The listing builds one solid part. Answer for the finished solid, in the listing's coordinates (mm). A direction names the side the tool comes from. Give positions to 0.01 mm unless a question says otherwise; leave off trailing zeros. Write each loop counter-clockwise with the first axis right and the second up, starting at its lowest first coordinate (ties: lowest second). Pieces come first, ordered by that corner, then holes. Notation, with made-up numbers: (61, 21) -> (78, 21) arc R29 cw to (78, 52) -> close; hole circle Ø10 at (-31.75, -18). An arc over 180 degrees is marked (long way). One line per question, with ' | ' between items.
from build123d import *

# Parameters (mm, degrees)
SKETCH1_W           = 35
SKETCH1_H           = 35
SKETCH1_W_2         = 31
SKETCH1_H_2         = 31
BOSS_EXTRUDE1_DEPTH = 360
SKETCH2_R           = 4
CUT_EXTRUDE1_DEPTH  = 364.386846212


with BuildPart() as part:
    # Sketch1 → Boss-Extrude1 (new body)
    with BuildSketch(Plane(origin=(0, 0, 0), x_dir=(0, 0, -1), z_dir=(1, 0, 0))):
        with Locations((17.5, 17.5)):
            Rectangle(SKETCH1_W, SKETCH1_H)
        with Locations((17.5, 17.5)):
            Rectangle(SKETCH1_W_2, SKETCH1_H_2, mode=Mode.SUBTRACT)
    extrude(amount=BOSS_EXTRUDE1_DEPTH)

    # Sketch2 → Cut-Extrude1 (cut, through all)
    with BuildSketch(Plane.XY):
        with Locations((330, 17.5)):
            Circle(SKETCH2_R)
        with Locations((230, 17.5)):
            Circle(SKETCH2_R)
    extrude(amount=-CUT_EXTRUDE1_DEPTH, mode=Mode.SUBTRACT)


solid = part.part
Item 1: Determine the mould class of faces 1 (the face through (177, 33, -17)), 2 (the face through (177, 17, -35)), 3 (the face through (226.004, 17.676, -33.986)), 4 (the face through (177, 0, -17)) for opening direction Y: pulls with the +Y half, pulls with the -Y half, needs draft (parallel to the pull), parting line crosses it, or undercut.
Answers below:
face 1: undercut | face 2: needs draft | face 3: undercut | face 4: pulls with the -Y half
Item 2: Consider line 1 (Z direction, x = 339, y = 9); line 2 (Y direction, x = 195.5, z = -30.5); line 3 (X direction, y = 17, z = -1). Determine where each line is inside the solid, lowest interval first. Write a range as [from, to].
Answers below:
line 1: [-35, -33], [-2, 0] | line 2: [0, 2], [33, 35] | line 3: [0, 226.03], [233.97, 326.03], [333.97, 360]
Item 3: Find section D-D (x = 230). Write down the section's boundary in (y, z), then the cut area to 3 significant figures.
Answers below:
outline: (0, -35) -> (13.5, -35) -> (13.5, -33) -> (2, -33) -> (2, -2) -> (13.5, -2) -> (13.5, 0) -> (0, 0) -> close; (21.5, -35) -> (35, -35) -> (35, 0) -> (21.5, 0) -> (21.5, -2) -> (33, -2) -> (33, -33) -> (21.5, -33) -> close | area: 232 mm²
Item 4: A flat-ended cylindrical pin translates along its axis: pin 1 (5 mm diameter, centred on x = 230, y = 17.5, fed in from -Z). Find the tip coordinate at first contact, or state that the pin passes through.
Answers below:
pin 1: through
Item 5: Find section C-C (x = 49). Write down the section's boundary in (y, z), then the cut area to 3 significant figures.
Answers below:
outline: (0, -35) -> (35, -35) -> (35, 0) -> (0, 0) -> close; hole (2, -33) -> (33, -33) -> (33, -2) -> (2, -2) -> close | area: 264 mm²
Item 6: Find section B-B (y = 25.5). Write down the section's boundary in (x, z).
Answers below:
outline: (0, -35) -> (360, -35) -> (360, -33) -> (0, -33) -> close; (0, -2) -> (360, -2) -> (360, 0) -> (0, 0) -> close
Item 7: A tool of negligible diameter and unlimited length cuts with its end or side. For faces 5 (the face through (177, 2, -17)), 6 (the face through (326.004, 17.676, -0.986)), from which of +Z, -Z, +X, -X, +Y, -Y can it reach the whole face along a straight path? Write none if from no direction.
Answers below:
face 5: +X, -X | face 6: +Z, -Z
Item 8: Find section A-A (z = -23). Write down the section's boundary in (x, y), then the cut area to 3 significant figures.
Answers below:
outline: (0, 0) -> (360, 0) -> (360, 2) -> (0, 2) -> close; (0, 33) -> (360, 33) -> (360, 35) -> (0, 35) -> close | area: 1,440 mm²
